Work out the finished part from the listing and answer in its coordinate system (mm). A direction names the side the tool comes from. Round coordinates to 2 decimals unless told otherwise and drop trailing zeros. Write each loop counter-clockwise with the first axis right and the second up, starting at its lowest first coordinate (ties: lowest second). Pieces come first, ordered by that corner, then holes. Notation, with made-up numbers: (-23.5, 18) - (-19.5, 18) arc R5 ccw to (-19.5, 23) - close; hole circle Ø10 at (36, 81). An arc over 180 degrees is marked (long way). Answer as a JSON object with one key per item and string values.
```python
from build123d import *

# Parameters (mm, degrees)
SKETCH1_R                    = 3.2
BASE_FLANGE1_DEPTH           = 1.5875
EDGE_FLANGE1_STRIP_W         = 7.8232
EDGE_FLANGE1_STRIP_H         = 1.5875
EDGE_FLANGE1_STRIP_CUT_DEPTH = 12
EDGE_FLANGE1_DEPTH           = 12
HOLE1_START                  = 25
HOLE1_OUTLINE_R              = 1.8288
HOLE1_DEPTH                  = 1.5875
FILLET1_RADIUS               = 6
FILLET1_LENGTH               = 1.5875


# Read off the part's stored shape, not the designer's step: Hole1
# Sheet-metal steps are written as plain solids
with BuildPart() as part:
    # Sketch1 → Base-Flange1 (new body)
    with BuildSketch(Plane(origin=(0, 0, 0), x_dir=(1, 0, 0), z_dir=(0, 1, 0))):
        with BuildLine():
            Line((0, 6), (25, 6))
            Line((25, 6), (25, -6))
            Line((25, -6), (0, -6))
            ThreePointArc((0, -6), (-6, 0), (0, 6))
        make_face()
        with Locations(Location((0, 0, 0), (0, 0, 270))):
            Circle(SKETCH1_R, mode=Mode.SUBTRACT)
    extrude(amount=BASE_FLANGE1_DEPTH)

    # Edge-Flange1 strip (across the edge) → Edge-Flange1 strip cut (cut)
    with BuildSketch(Plane(origin=(25, 1.5875, 6), x_dir=(-1, 0, 0), z_dir=(0, 0, -1))):
        with Locations((-3.175, -0.79375)):
            Rectangle(EDGE_FLANGE1_STRIP_W, EDGE_FLANGE1_STRIP_H)
    extrude(amount=EDGE_FLANGE1_STRIP_CUT_DEPTH, mode=Mode.SUBTRACT)

    # Edge-Flange1 section (across the edge) → Edge-Flange1 (add)
    with BuildSketch(Plane(origin=(25, 1.5875, 6), x_dir=(-1, 0, 0), z_dir=(0, 0, -1))):
        with BuildLine():
            Line((-1.5875, 0.7366), (-1.5875, 12.7))
            Line((-1.5875, 12.7), (0, 12.7))
            Line((0, 12.7), (0, 0.7366))
            ThreePointArc((0, 0.7366), (0.215745145, 0.215745145), (0.7366, 0))
            Line((0.7366, 0), (0.7366, -1.5875))
            ThreePointArc((0.7366, -1.5875), (-0.90678687, -0.90678687), (-1.5875, 0.7366))
        make_face()
    extrude(amount=EDGE_FLANGE1_DEPTH)

    # Hole1 outline → Hole1 (cut)
    with BuildSketch(Plane.YZ.offset(HOLE1_START)):
        with Locations((7.9375, 0)):
            Circle(HOLE1_OUTLINE_R)
    extrude(amount=HOLE1_DEPTH, mode=Mode.SUBTRACT)

    # Fillet1: full round fillet: the end face becomes a half cylinder, R = half its width
    fillet1_face = Plane((25.79375, 14.2875, 0), x_dir=(1, 0, 0), z_dir=(0, 1, 0))  # on the end face: x along it, z out of the body
    fillet1_slab = fillet1_face.offset(-FILLET1_RADIUS / 2) * Box(FILLET1_LENGTH, 2 * FILLET1_RADIUS, FILLET1_RADIUS, mode=Mode.PRIVATE)  # the body's end, R deep
    fillet1_round = Plane((25.79375, 8.2875, 0), x_dir=(0, 1, 0), z_dir=(1, 0, 0)) * Cylinder(FILLET1_RADIUS, FILLET1_LENGTH, mode=Mode.PRIVATE)  # its axis R under the face
    add(fillet1_slab - fillet1_round, mode=Mode.SUBTRACT)


solid = part.part
```
Item 1: A cutting plane is placed at D-D (y = 7.75). Write down the section's boundary in (x, z), and give its area (3 significant figures).
Results found:
{"outline": "(25, -6) - (26.59, -6) - (26.59, -1.82) - (25, -1.82) - close; (25, 1.82) - (26.59, 1.82) - (26.59, 6) - (25, 6) - close", "area": "13.3 mm²"}
Item 2: Determine the mould class of faces 1 (the cylindrical face through (-1.947, 0.783, -2.539)), 2 (the flat face through (16, 1, -6)), 3 (the flat face through (9, 1.588, 0)) for opening direction Z: pulls with the +Z half, pulls with the -Z half, needs draft (parallel to the pull), parting line crosses it, or undercut.
Results found:
{"face 1": "undercut", "face 2": "pulls with the -Z half", "face 3": "needs draft"}
Item 3: Consider line 1 along X through (y, z) = (5.5, -0.5); line 2 along X through (y, z) = (0.95, 0); line 3 along Y through (x, z) = (5.5, 3). Determine where each line is inside the solid, lowest interval first.
Results found:
{"line 1": "25 to 26.59", "line 2": "-6 to -3.2, 3.2 to 26.14", "line 3": "0 to 1.59"}
Item 4: A cutting plane is placed at C-C (x = 16.5). Write down the section's boundary in (y, z).
Results found:
{"outline": "(0, -6) - (1.59, -6) - (1.59, 6) - (0, 6) - close"}
Item 5: A cutting plane is placed at A-A (z = 0). Write down the section's boundary in (x, y).
Results found:
{"outline": "(-6, 0) - (-3.2, 0) - (-3.2, 1.59) - (-6, 1.59) - close; (3.2, 0) - (24.26, 0) arc R2.32 ccw to (26.59, 2.32) - (26.59, 6.11) - (25, 6.11) - (25, 2.32) arc R0.74 cw to (24.26, 1.59) - (3.2, 1.59) - close; (25, 9.77) - (26.59, 9.77) - (26.59, 14.29) - (25, 14.29) - close"}
Item 6: A cutting plane is placed at B-B (y = 9.25). Write down the section's boundary in (x, z), and give its area (3 significant figures).
Results found:
{"outline": "(25, -5.92) - (26.59, -5.92) - (26.59, -1.27) - (25, -1.27) - close; (25, 1.27) - (26.59, 1.27) - (26.59, 5.92) - (25, 5.92) - close", "area": "14.8 mm²"}
Item 7: Each of these flat-tipped pins is pushed along its axis until it touches: P1, Ø6, axis at y = 7.94, z = 0, coming from the -X side; P2, Ø5, axis at x = -1, z = 3.5, coming from the +Y side. Where does it stop, or does it pass through?
Results found:
{"P1": "x = 25", "P2": "y = 1.59"}
Item 8: For faces 4 (the flat face through (9, 0, 0)), 5 (the flat face through (25, 5.7, 0.1)), determine the directions among +Z, -Z, +X, -X, +Y, -Y from which every point of the face is accessible in a straight line to the end or side of a thin tool.
Results found:
{"face 4": "+Z, -Z, +X, -X, -Y", "face 5": "+Z, -Z, -X, +Y"}
